Build history of the part. All positions in model axes, mm. A direction names the side the tool comes from. Coordinates: 2 decimals unless noted, no trailing zeros. Loops run counter-clockwise (first coordinate to the right, second up) from the corner with the lowest first, then second, coordinate; pieces in that order, holes last.
Item 1: 3-axis set-ups, long thin cutter, end or side, ignore diameter. For faces 1 (the face through (4.62, 2.18, -1.39)), 2 (the face through (2.958, 1.205, 5.817)), 3 (the face through (2.958, -4.407, 4.022)), 4 (the face through (2.96, 5.13, 3)): which of +Z, -Z, +X, -X, +Y, -Y reach the whole face in a straight line?
Item 2: Drill centre lines: line 1 along Z through (x, y) = (5.25, -5); line 2 along Y through (x, z) = (-3.5, 0) (3 decimals); line 3 along Y through (x, z) = (2.25, 5.25). Where is each one in solid material? Low to high.
Item 3: Mould opens along X. For faces 5 (the face through (2.96, -0.52, 4.97)), 6 (the face through (3.2, -3, 0)) say: released by +X, released by -X, zero draft, split by the parting line, or undercut.
Item 4: Cut at A-A (x = -2.25). List the corners of the cut face in (y, z) (3 decimals).
from build123d import *

# Parameters (mm, degrees)
BASPROSKE_W             = 6
BASPROSKE_H             = 6.8
TOOTHCUT_DEPTH          = 12.334901852
TEETHCUTS_COUNT         = 15
TEETHCUTS_ANGLE         = 336
BORSKE_R                = 0.4
BORE_DEPTH              = 50.0000508
ESQUISSE1_R             = 4.5
BOSS_EXTRU_1_DEPTH      = 6
ENL_V_MAT_EXTRU_1_REACH = 17.369
ESQUISSE2_R             = 1.585
ESQUISSE3_R             = 4.085
ESQUISSE3_R_2           = 2.585
ENL_V_MAT_EXTRU_2_DEPTH = 2.8
CHANFREIN1_SIZE         = 0.25


with BuildPart() as part:
    # BasProSke → Base-Revolve (revolve)
    with BuildSketch(Plane(origin=(0, 0, 0), x_dir=(1, 0, 0), z_dir=(0, 1, 0)), mode=Mode.PRIVATE) as base_revolve_sk:
        with Locations((3, 3.4)):
            Rectangle(BASPROSKE_W, BASPROSKE_H)
    revolve(base_revolve_sk.sketch.rotate(Axis((-10, 0, 0), (1, 0, 0)), 180), axis=Axis((-10, 0, 0), (1, 0, 0)))

    # TooCutSke → ToothCut (cut, through all)
    with BuildSketch(Plane(origin=(0, 0, 0), x_dir=(0, 0, -1), z_dir=(1, 0, 0))):
        with BuildLine():
            ThreePointArc((0.424668738, 4.980929377), (0, 4.999), (-0.424668738, 4.980929377))
            ThreePointArc((-0.424668738, 4.980929377), (-0.664927989, 5.931738726), (-1.265455885, 6.70706393))
            ThreePointArc((-1.265455885, 6.70706393), (0, 6.8254), (1.265455885, 6.70706393))
            ThreePointArc((1.265455885, 6.70706393), (0.664927989, 5.931738726), (0.424668738, 4.980929377))
        make_face()
    toothcut = extrude(amount=TOOTHCUT_DEPTH, mode=Mode.SUBTRACT)

    # TeethCuts: ToothCut ×15 about axis
    teethcuts_axis = Axis((-10, 0, 0), (1, 0, 0))
    for i in range(1, TEETHCUTS_COUNT):
        add(toothcut.rotate(teethcuts_axis, i * TEETHCUTS_ANGLE / (TEETHCUTS_COUNT - 1)), mode=Mode.SUBTRACT)

    # BorSke → Bore (cut, symmetric)
    with BuildSketch(Plane(origin=(0, 0, 0), x_dir=(0, 0, -1), z_dir=(1, 0, 0))):
        with Locations(Location((0, 0, 0), (0, 0, 180))):
            Circle(BORSKE_R)
    extrude(amount=BORE_DEPTH, both=True, mode=Mode.SUBTRACT)

    # Esquisse1 → Boss.-Extru.1 (add)
    with BuildSketch(Plane.ZY):
        with Locations(Location((0, 0, 0), (0, 0, 180))):
            Circle(ESQUISSE1_R)
    extrude(amount=BOSS_EXTRU_1_DEPTH)

    # Esquisse2 → Enlèv. mat.-Extru.1 (cut, up to next)
    with BuildSketch(Plane.ZY.offset(6), mode=Mode.PRIVATE) as enl_v_mat_extru_1_sk1:
        Circle(ESQUISSE2_R)
    enl_v_mat_extru_1_tool1 = extrude(enl_v_mat_extru_1_sk1.sketch, amount=-ENL_V_MAT_EXTRU_1_REACH, mode=Mode.PRIVATE) & part.part
    add(enl_v_mat_extru_1_tool1.solids().sort_by_distance((-6, 0, 0))[0], mode=Mode.SUBTRACT)

    # Esquisse3 → Enlèv. mat.-Extru.2 (cut)
    with BuildSketch(Plane(origin=(6, 0, 0), x_dir=(0, 0, -1), z_dir=(1, 0, 0))):
        Circle(ESQUISSE3_R)
        Circle(ESQUISSE3_R_2, mode=Mode.SUBTRACT)
    extrude(amount=-ENL_V_MAT_EXTRU_2_DEPTH, mode=Mode.SUBTRACT)

    # Chanfrein1
    chanfrein1_edges = [part.edges().sort_by_distance(p)[0] for p in [
        (-6, 0, 4.5),
    ]]
    chamfer(chanfrein1_edges, length=CHANFREIN1_SIZE)


solid = part.part
Filled sheet:
1. face 1: +X
1. face 2: +X, -X
1. face 3: +X, -X, -Y
1. face 4: +X, -X, +Y
2. line 1: z = -2.91 to -1.52, -0.63 to 0.63, 1.52 to 2.91
2. line 2: y = -4.5 to -1.585, 1.585 to 4.5
2. line 3: y = -2.36 to -1.02, -0.1 to 1.21, 2.3 to 3.55
3. face 5: zero draft
3. face 6: released by +X
4. outline: circle Ø9 at (0, 0); hole circle Ø3.17 at (0, 0)
